Could you check a few things on this drawing? It's one solid part, dimensions in mm from its lowest x, y, z. Round coordinates to 2 decimals unless told otherwise and drop trailing zeros. Write each loop counter-clockwise with the first axis right and the second up, starting at its lowest first coordinate (ties: lowest second). Pieces come first, ordered by that corner, then holes. Notation, with made-up numbers: (23, 5.25) -> (27, 5.25) arc R23 cw to (27, 24.25) -> close; hole circle Ø10 at (26.25, 82.5). An arc over 180 degrees is marked (long way). Answer in a Markdown table with one row per item. Add a question column.
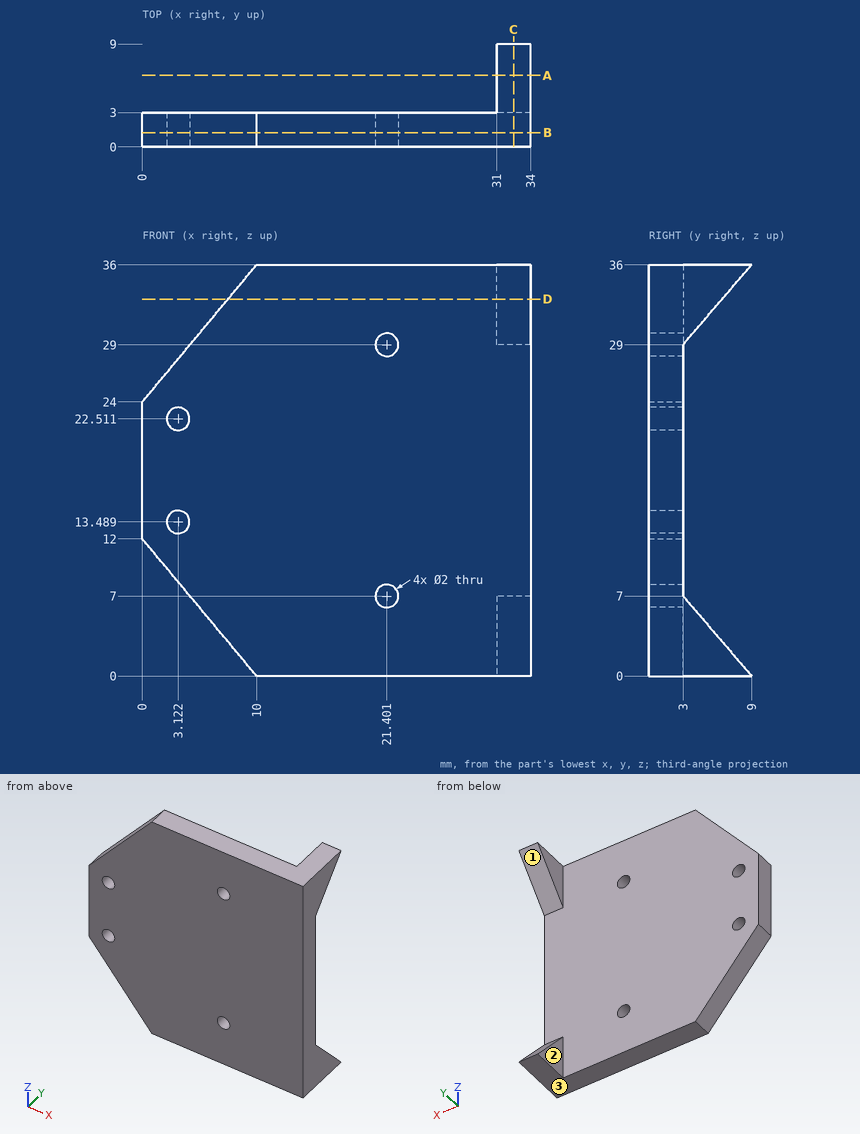
(1) If we mould it in two halves opening along Z, with no side actions, what happens to the marked faces 1, 2 and 3? For each: pulls with the +Z half, pulls with the -Z half, needs draft (parallel to the pull), parting line crosses it, or undercut.
(2) Suppose I cut it at C-C, the plane x = 32.5. Please give me the cut outline in (y, z).
(3) Suppose I cut it at B-B, the plane y = 1.25. Please give me the cut outline in (x, z), then the cut area to 3 significant figures.
(4) Suppose I cut it at D-D, the plane z = 33. Please give me the cut outline in (x, y).
(5) For P1, Ø3, axis at x = 3.12, z = 22.51, coming from the +Y side; P2, Ø5, axis at y = 1.5, z = 24, coming from the -X side; P3, Ø3, axis at y = 5, z = 9.5, coming from the +X side; P4, Ø3, axis at y = 6.5, z = 2, coming from the -X side, each with a flat end and sliding along its axis, tell me the tip position at first contact or that it passes through.
(6) I need wall thicknesses on L1, parallel to Y at x = 28, z = 33.5; L2, parallel to Z at x = 22, y = 1.25; L3, parallel to X at y = 0.6, z = 29 (1 decimal). Which ranges of each line are inside material? Lowest first, please.
(7) Suppose I cut it at A-A, the plane y = 6.25. Please give me the cut outline in (x, z).
Response:
| question | item | result |
|---|---|---|
| 1 | face 1 | undercut |
| 1 | face 2 | needs draft |
| 1 | face 3 | pulls with the -Z half |
| 2 | outline | (0, 0) -> (9, 0) -> (3, 7) -> (3, 29) -> (9, 36) -> (0, 36) -> close |
| 3 | outline | (0, 12) -> (10, 0) -> (34, 0) -> (34, 36) -> (10, 36) -> (0, 24) -> close; hole circle Ø2 at (3.12, 13.49); hole circle Ø2 at (3.12, 22.51); hole circle Ø2 at (21.4, 7); hole circle Ø2 at (21.4, 29) |
| 3 | area | 1,090 mm² |
| 4 | outline | (7.5, 0) -> (34, 0) -> (34, 6.43) -> (31, 6.43) -> (31, 3) -> (7.5, 3) -> close |
| 5 | P1 | y = 3 |
| 5 | P2 | x = 0 |
| 5 | P3 | through |
| 5 | P4 | x = 31 |
| 6 | L1 | 0 to 3 |
| 6 | L2 | 0 to 6.2, 7.8 to 28.2, 29.8 to 36 |
| 6 | L3 | 4.2 to 20.4, 22.4 to 34 |
| 7 | outline | (31, 0) -> (34, 0) -> (34, 3.21) -> (31, 3.21) -> close; (31, 32.79) -> (34, 32.79) -> (34, 36) -> (31, 36) -> close |
